The model under review builds one solid part; all positions refer to its coordinate system, in mm. A direction names the side the tool comes from. Round coordinates to 2 decimals unless told otherwise and drop trailing zeros. Write each loop counter-clockwise with the first axis right and the second up, starting at its lowest first coordinate (ties: lowest second). Pieces come first, ordered by that corner, then holes. Notation, with made-up numbers: (-20.75, -34.75) -> (23.25, -34.75) arc R21 cw to (23.25, -15.75) -> close; hole circle Ø8 at (63, 32). An arc over 180 degrees is marked (long way). Answer as a JSON object with one key per item and string values. Group by question number.
1) We need section B-B, the plane z = 1.9. Write out the cut boundary in (x, y), then the cut area to 3 significant figures.
2) Machinability: for faces 1 (the flat face through (12.8, 17, 2)), 2 (the flat face through (7, 17, 1)), which of the approach directions +Z, -Z, +X, -X, +Y, -Y give a long, thin tool a straight path to every point of the face, cutting with its end or side? Answer none if there is none.
3) To check wall thickness, follow probe 1 along Z at (x, y) = (3.5, 11.5); probe 2 along Y at (x, z) = (12.75, 1.45); probe 3 along X at (y, z) = (16.5, 2.2). State the ranges of each line that lie inside material, in increasing order. Write a range as [from, to].
4) We need section C-C, the plane y = 16.25. Write out the cut boundary in (x, z).
5) Mouldability with a two-part tool opening along Y and no side actions: class faces 3 (the flat face through (7, 17, 2.26)), 4 (the flat face through (13, 17, 2)) as pulls with the +Y half, pulls with the -Y half, needs draft (parallel to the pull), parting line crosses it, or undercut.
6) We need section A-A, the plane x = 4.25. Write out the cut boundary in (y, z).
from build123d import *

# Parameters (mm, degrees)
SKETCH011_W    = 11.5
SKETCH011_H    = 12
PAD008_DEPTH   = 1.46
FILLET003_R    = 0.4
THICKNESS003_T = -0.2


with BuildPart() as part:
    # Sketch011 (on Face1 of ReferenceLinearPattern004004) → Pad008 (new body)
    with BuildSketch(Plane.XY.offset(1)):
        with Locations((7.25, 16.7)):
            Rectangle(SKETCH011_W, SKETCH011_H)
    extrude(amount=PAD008_DEPTH)

    # Fillet003
    fillet003_edges = [part.edges().sort_by_distance(p)[0] for p in [
        (7.25, 10.7, 2.46),
        (7.25, 10.7, 1),
        (7.25, 22.7, 2.46),
        (7.25, 22.7, 1),
    ]]
    fillet(fillet003_edges, radius=FILLET003_R)

    # Thickness003
    thickness003_openings = [part.faces().sort_by_distance(p)[0] for p in [
        (1.5, 16.7, 1.73),
    ]]
    offset(amount=THICKNESS003_T, openings=thickness003_openings)


solid = part.part
Here are the results:
{
 "1": {"outline": "(1.5, 10.7) -> (13, 10.7) -> (13, 22.7) -> (1.5, 22.7) -> (1.5, 22.5) -> (12.8, 22.5) -> (12.8, 10.9) -> (1.5, 10.9) -> close", "area": "6.92 mm^2"},
 "2": {"face 1": "-X", "face 2": "-Z, +X, -X, +Y, -Y"},
 "3": {"probe 1": "z = [1, 1.2], [2.26, 2.46]", "probe 2": "y = [10.7, 10.9], [22.5, 22.7]", "probe 3": "x = [12.8, 13]"},
 "4": {"outline": "(1.5, 1) -> (13, 1) -> (13, 2.46) -> (1.5, 2.46) -> (1.5, 2.26) -> (12.8, 2.26) -> (12.8, 1.2) -> (1.5, 1.2) -> close"},
 "5": {"face 3": "undercut", "face 4": "needs draft"},
 "6": {"outline": "(10.7, 1.4) arc R0.4 ccw to (11.1, 1) -> (22.3, 1) arc R0.4 ccw to (22.7, 1.4) -> (22.7, 2.06) arc R0.4 ccw to (22.3, 2.46) -> (11.1, 2.46) arc R0.4 ccw to (10.7, 2.06) -> close; hole (10.9, 1.4) arc R0.2 ccw to (11.1, 1.2) -> (22.3, 1.2) arc R0.2 ccw to (22.5, 1.4) -> (22.5, 2.06) arc R0.2 ccw to (22.3, 2.26) -> (11.1, 2.26) arc R0.2 ccw to (10.9, 2.06) -> close"}
}
